```python
from build123d import *

# Parameters (mm, degrees)
F0_W     = 68
F0_H     = 12
F0_W_2   = 5
F0_H_2   = 14
F1_DEPTH = 1.6
F4_R     = 0.35
F5_R     = 0.35
F6_R     = 0.35
F2_R     = 0.35
F7_DEPTH = 4
F8_R     = 1.1
F9_DEPTH = 25


with BuildPart() as f1:
    # F0 (on Top) → F1 (new body)
    with BuildSketch(Plane.XY):
        with Locations((41.3172904253, 1.6970097786)):
            Rectangle(F0_W, F0_H)
        with Locations((4.8172904253, 14.6970097786)):
            Rectangle(F0_W_2, F0_H_2)
        with Locations((41.3172904253, 14.6970097786)):
            Rectangle(F0_W, F0_H_2)
        with Locations((77.8172904253, 14.6970097786)):
            Rectangle(F0_W_2, F0_H_2)
        with Locations((41.3172904253, 27.6970097786)):
            Rectangle(F0_W, F0_H)
    extrude(amount=F1_DEPTH)

    # F4 (on face) + F5 (on face) + F6 (on face) + F3 (on face) + F2 (on face) → F7 (cut)
    with BuildSketch(Plane.XY.offset(1.6)):
        with Locations((51.6172904253, 6.6970097786)):
            Circle(F4_R)
        with Locations((56.6172904253, 6.6970097786)):
            Circle(F4_R)
        with Locations((54.1172904253, 6.6970097786)):
            Circle(F4_R)
    with BuildSketch(Plane.XY.offset(1.6)):
        with Locations((28.0672904253, -1.3029902214)):
            Circle(F5_R)
        with Locations((30.5672904253, -1.3029902214)):
            Circle(F5_R)
        with Locations((52.0672904253, -1.3029902214)):
            Circle(F5_R)
        with Locations((54.5672904253, -1.3029902214)):
            Circle(F5_R)
        with Locations((54.5672904253, 30.6970097786)):
            Circle(F5_R)
        with Locations((52.0672904253, 30.6970097786)):
            Circle(F5_R)
        with Locations((30.5672904253, 30.6970097786)):
            Circle(F5_R)
        with Locations((28.0672904253, 30.6970097786)):
            Circle(F5_R)
    with BuildSketch(Plane.XY.offset(1.6)):
        with Locations((27.5672904253, 6.6970097786)):
            Circle(F6_R)
        with Locations((31.0672904253, 6.6970097786)):
            Circle(F6_R)
    with BuildSketch(Plane.XY.offset(1.6)):
        with BuildLine():
            Line((54.8172904253, 15.4470097786), (53.8172904253, 15.4470097786))
            ThreePointArc((53.8172904253, 15.4470097786), (53.640513733, 15.5202330803), (53.5672904253, 15.6970097701))
            ThreePointArc((53.5672904253, 15.6970097701), (54.3172904296, 14.9470097786), (55.0672904253, 15.6970097786))
            ThreePointArc((55.0672904253, 15.6970097786), (54.9940671206, 15.5202330833), (54.8172904253, 15.4470097786))
        make_face()
        with BuildLine():
            ThreePointArc((53.5672904253, 15.6970097701), (53.640513733, 15.5202330803), (53.8172904253, 15.4470097786))
            Line((53.8172904253, 15.4470097786), (54.8172904253, 15.4470097786))
            ThreePointArc((54.8172904253, 15.4470097786), (54.9940671206, 15.5202330833), (55.0672904253, 15.6970097786))
            ThreePointArc((55.0672904253, 15.6970097786), (54.9940671206, 15.8737864739), (54.8172904253, 15.9470097786))
            Line((54.8172904253, 15.9470097786), (53.8172904253, 15.9470097786))
            ThreePointArc((53.8172904253, 15.9470097786), (53.640513727, 15.8737864709), (53.5672904253, 15.6970097701))
        make_face()
        with BuildLine():
            ThreePointArc((55.0672904253, 15.6970097786), (54.317290421, 16.4470097786), (53.5672904253, 15.6970097701))
            ThreePointArc((53.5672904253, 15.6970097701), (53.640513727, 15.8737864709), (53.8172904253, 15.9470097786))
            Line((53.8172904253, 15.9470097786), (54.8172904253, 15.9470097786))
            ThreePointArc((54.8172904253, 15.9470097786), (54.9940671206, 15.8737864739), (55.0672904253, 15.6970097786))
        make_face()
        with BuildLine():
            Line((51.1672904253, 13.7970097786), (51.8672904253, 13.7970097786))
            ThreePointArc((51.8672904253, 13.7970097786), (52.0440671206, 13.7237864739), (52.1172904253, 13.5470097786))
            ThreePointArc((52.1172904253, 13.5470097786), (51.5172904253, 14.1470097786), (50.9172904253, 13.5470097786))
            ThreePointArc((50.9172904253, 13.5470097786), (50.99051373, 13.7237864739), (51.1672904253, 13.7970097786))
        make_face()
        with BuildLine():
            ThreePointArc((52.1172904253, 13.5470097786), (52.0440671206, 13.7237864739), (51.8672904253, 13.7970097786))
            Line((51.8672904253, 13.7970097786), (51.1672904253, 13.7970097786))
            ThreePointArc((51.1672904253, 13.7970097786), (50.99051373, 13.7237864739), (50.9172904253, 13.5470097786))
            ThreePointArc((50.9172904253, 13.5470097786), (50.99051373, 13.3702330833), (51.1672904253, 13.2970097786))
            Line((51.1672904253, 13.2970097786), (51.8672904253, 13.2970097786))
            ThreePointArc((51.8672904253, 13.2970097786), (52.0440671206, 13.3702330833), (52.1172904253, 13.5470097786))
        make_face()
        with BuildLine():
            ThreePointArc((50.9172904253, 13.5470097786), (51.5172904253, 12.9470097786), (52.1172904253, 13.5470097786))
            ThreePointArc((52.1172904253, 13.5470097786), (52.0440671206, 13.3702330833), (51.8672904253, 13.2970097786))
            Line((51.8672904253, 13.2970097786), (51.1672904253, 13.2970097786))
            ThreePointArc((51.1672904253, 13.2970097786), (50.99051373, 13.3702330833), (50.9172904253, 13.5470097786))
        make_face()
        with BuildLine():
            Line((56.7672904253, 13.2970097786), (57.4672904253, 13.2970097786))
            ThreePointArc((57.4672904253, 13.2970097786), (57.6440671206, 13.3702330833), (57.7172904253, 13.5470097786))
            ThreePointArc((57.7172904253, 13.5470097786), (57.6440671206, 13.7237864739), (57.4672904253, 13.7970097786))
            Line((57.4672904253, 13.7970097786), (56.7672904253, 13.7970097786))
            ThreePointArc((56.7672904253, 13.7970097786), (56.59051373, 13.7237864739), (56.5172904253, 13.5470097786))
            ThreePointArc((56.5172904253, 13.5470097786), (56.59051373, 13.3702330833), (56.7672904253, 13.2970097786))
        make_face()
        with BuildLine():
            ThreePointArc((57.7172904253, 13.5470097786), (57.6440671206, 13.3702330833), (57.4672904253, 13.2970097786))
            Line((57.4672904253, 13.2970097786), (56.7672904253, 13.2970097786))
            ThreePointArc((56.7672904253, 13.2970097786), (56.59051373, 13.3702330833), (56.5172904253, 13.5470097786))
            ThreePointArc((56.5172904253, 13.5470097786), (57.1172904253, 12.9470097786), (57.7172904253, 13.5470097786))
        make_face()
        with BuildLine():
            ThreePointArc((57.4672904253, 13.7970097786), (57.6440671206, 13.7237864739), (57.7172904253, 13.5470097786))
            ThreePointArc((57.7172904253, 13.5470097786), (57.1172904253, 14.1470097786), (56.5172904253, 13.5470097786))
            ThreePointArc((56.5172904253, 13.5470097786), (56.59051373, 13.7237864739), (56.7672904253, 13.7970097786))
            Line((56.7672904253, 13.7970097786), (57.4672904253, 13.7970097786))
        make_face()
    with BuildSketch(Plane.XY.offset(1.6)):
        with Locations((27.3172904253, 14.6970097786)):
            Circle(F2_R)
        with Locations((29.3172904253, 14.6970097786)):
            Circle(F2_R)
        with Locations((31.3172904253, 14.6970097786)):
            Circle(F2_R)
    extrude(amount=-F7_DEPTH, mode=Mode.SUBTRACT)

    # F8 (on face) → F9 (cut)
    with BuildSketch(Plane.XY.offset(1.6)):
        with Locations((62.3172904253, 26.6970097786)):
            Circle(F8_R)
        with Locations((20.3172904253, 26.6970097786)):
            Circle(F8_R)
        with Locations((68.3172904253, 2.6970097786)):
            Circle(F8_R)
        with Locations((14.3172904253, 2.6970097786)):
            Circle(F8_R)
    extrude(amount=-F9_DEPTH, mode=Mode.SUBTRACT)


solid = f1.part
```
Geometry check sheet. Reference: the model listing, model coordinates, mm. A direction names the side the tool comes from. Round coordinates to 2 decimals unless told otherwise and drop trailing zeros. Loops run counter-clockwise (first coordinate to the right, second up) from the corner with the lowest first, then second, coordinate; pieces in that order, holes last. Notation, with made-up numbers: M 48.5,-18 L 98.5,-18 A16 cw 98.5,-4 Z; hole C -29.75,33.25 d8. An arc over 180 degrees is marked long. Return JSON: item names as keys, results as strings. Group by question number.
(1) Set-up check for faces 1 (the face through (75.317, 28, 1)), 2 (the face through (5, 7.697, 1)), 3 (the face through (7.317, 28, 1)), 4 (the face through (67.22, 2.75, 0.81)): record each of +Z, -Z, +X, -X, +Y, -Y from which the full face is reachable in a straight line by a thin tool's end or side.
(2) Section check A-A, the plane y = 24.5. Enter the section's corners in (x, z), and give its area (3 significant figures).
(3) Scan lines: line 1 along Y through (x, z) = (77, 0.25); line 2 along X through (y, z) = (-1.5, 0.5); line 3 along X through (y, z) = (28.5, 0.5). Record each from-to range of solid material in increasing order. Write a range as [from, to].
(4) Section check B-B, the plane z = 0.4. Give the number of separate pieces and of enclosed holes in the cut face, and give its area (3 significant figures).
(5) Mould release check, pull along Y, two halves, no side actions. Record for faces 5 (the face through (61.22, 26.75, 0.81)), 6 (the face through (75.317, 2, 1)), 7 (the face through (78, 21.697, 1)), 8 (the face through (78, 7.697, 1)): pulls with the +Y half, pulls with the -Y half, needs draft (parallel to the pull), parting line crosses it, or undercut.
(6) Go/stop test with flat-tipped pins: pin 1 (0.8 mm diameter, centred on y = 25, z = 1, fed in from -X); pin 2 (1.7 mm diameter, centred on x = 54.32, y = 15.7, fed in from -Z); pin 3 (0.8 mm diameter, centred on y = 3.5, z = 1, fed in from +X); pin 4 (0.8 mm diameter, centred on x = 5.5, z = 0.5, fed in from -Y). Record where each tip stops, or that it passes through.
Data:
{
 "1": {"face 1": "+Z, -Z, +X, +Y", "face 2": "+Z, -Z, -X, -Y", "face 3": "+Z, -Z, -X, +Y", "face 4": "+Z, -Z"},
 "2": {"outline": "M 7.32,0 L 75.32,0 L 75.32,1.6 L 7.32,1.6 Z", "area": "109 mm²"},
 "3": {"line 1": "[7.7, 21.7]", "line 2": "[7.32, 27.78], [28.36, 30.28], [30.86, 51.78], [52.36, 54.28], [54.86, 75.32]", "line 3": "[7.32, 75.32]"},
 "4": {"separate pieces": "1", "enclosed holes": "23", "area": "2,700 mm²"},
 "5": {"face 5": "undercut", "face 6": "needs draft", "face 7": "pulls with the +Y half", "face 8": "pulls with the -Y half"},
 "6": {"pin 1": "x = 7.32", "pin 2": "z = 0", "pin 3": "x = 75.32", "pin 4": "y = 7.7"}
}
